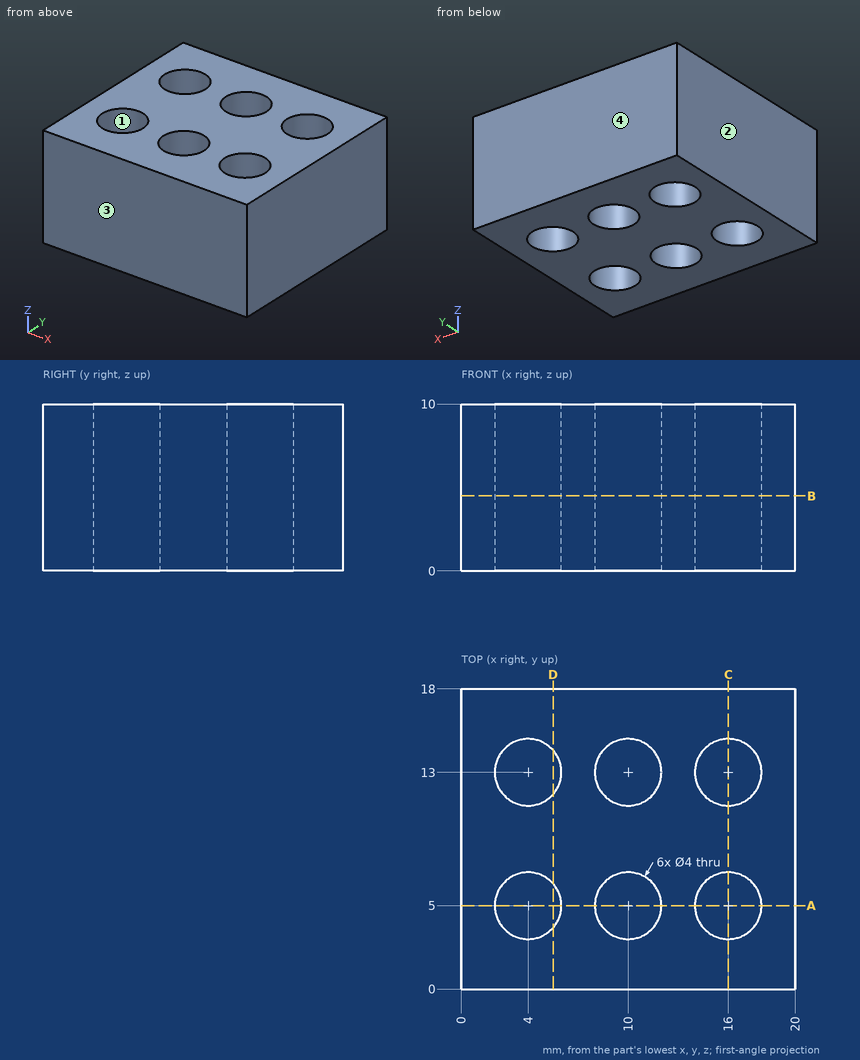
Geometry check sheet. Reference: drawing and pictorial views, mm from the part's lowest x, y, z. Round coordinates to 2 decimals unless told otherwise and drop trailing zeros. Loops run counter-clockwise (first coordinate to the right, second up) from the corner with the lowest first, then second, coordinate; pieces in that order, holes last. Notation, with made-up numbers: (39, 51) - (58, 51) arc R13 ccw to (58, 69) - close; hole circle Ø4 at (25.5, -8). An arc over 180 degrees is marked (long way). One line per question, with ' | ' between items. Start each with the question number.
1. Cross-section at C-C on x = 16. Record the cut outline in (y, z), then the cut area to 3 significant figures.
2. Scan lines: line 1 (Y direction, x = 4, z = 6.75); line 2 (Y direction, x = 11.75, z = 3); line 3 (X direction, y = 12.5, z = 5.25). Record each from-to range of solid material in increasing order. Write a range as [from, to].
3. Draft check along Y on the marked faces 1, 2, 3 and 4. Enter one of: released by +Y, released by -Y, zero draft, split by the parting line, or undercut.
4. Cross-section at D-D on x = 5.5. Record the cut outline in (y, z).
5. Cross-section at B-B on z = 4.5. Record the cut outline in (x, y), then the cut area to 3 significant figures.
6. Cross-section at A-A on y = 5. Record the cut outline in (x, z), then the cut area to 3 significant figures.
Taken from the geometry:
1) outline: (0, 0) - (3, 0) - (3, 10) - (0, 10) - close; (7, 0) - (11, 0) - (11, 10) - (7, 10) - close; (15, 0) - (18, 0) - (18, 10) - (15, 10) - close | area: 100 mm²
2) line 1: [0, 3], [7, 11], [15, 18] | line 2: [0, 4.03], [5.97, 12.03], [13.97, 18] | line 3: [0, 2.06], [5.94, 8.06], [11.94, 14.06], [17.94, 20]
3) face 1: undercut | face 2: zero draft | face 3: released by -Y | face 4: released by +Y
4) outline: (0, 0) - (3.68, 0) - (3.68, 10) - (0, 10) - close; (6.32, 0) - (11.68, 0) - (11.68, 10) - (6.32, 10) - close; (14.32, 0) - (18, 0) - (18, 10) - (14.32, 10) - close
5) outline: (0, 0) - (20, 0) - (20, 18) - (0, 18) - close; hole circle Ø4 at (4, 5); hole circle Ø4 at (4, 13); hole circle Ø4 at (10, 5); hole circle Ø4 at (10, 13); hole circle Ø4 at (16, 5); hole circle Ø4 at (16, 13) | area: 285 mm²
6) outline: (0, 0) - (2, 0) - (2, 10) - (0, 10) - close; (6, 0) - (8, 0) - (8, 10) - (6, 10) - close; (12, 0) - (14, 0) - (14, 10) - (12, 10) - close; (18, 0) - (20, 0) - (20, 10) - (18, 10) - close | area: 80.0 mm²
